from build123d import *

# Parameters (mm, degrees)
F1_DEPTH = 3.175
F3_DEPTH = 12.7
F5_R     = 1.27
F7_DEPTH = 38.1
F9_DEPTH = 57.1826710194


# Not quite as in the source:
# - a length typed as a fraction of an inch, garbled in the dataset ("3 / 203.2 mm" for 3/8 in), is restored


with BuildPart() as f1:
    # F0 (on Top) → F1 (new body)
    with BuildSketch(Plane.XY):
        Polygon((-63.5, -25.4), (63.5, -12.7), (63.5, 12.7), (-63.5, 25.4), align=None)
    extrude(amount=F1_DEPTH)

    # F2 (on Top) → F3 (join)
    with BuildSketch(Plane.XY):
        Polygon((-63.5, -25.4), (-63.5, -28.5908355097), (63.8159243079, -15.8592430789), (63.5, -12.7), align=None)
    extrude(amount=F3_DEPTH)

    # F4: F1 across plane


with BuildPart() as f1_1:
    add(f1.part)
    add(f1.part.mirror(Plane.XZ))

    # F5
    f5_edges = [f1_1.edges().sort_by_distance(p)[0] for p in [
        (0, -19.05, 3.175),
        (0, 19.05, 3.175),
    ]]
    fillet(f5_edges, radius=F5_R)

    # F6 (on face) → F7 (join)
    with BuildSketch(Plane(origin=(-63.5, 0, 0), x_dir=(0, -1, 0), z_dir=(-1, 0, 0))):
        Polygon((-25.4, 12.7), (-28.5908355097, 12.7), (-28.5908355097, 0), (-25.4, 0), (-25.4, 4.445), align=None)
        Polygon((25.4, 4.445), (25.4, 0), (28.5908355097, 0), (28.5908355097, 12.7), (25.4, 12.7), align=None)
    extrude(amount=F7_DEPTH)

    # F8 (on face) → F9 (cut, through all)
    with BuildSketch(Plane.XZ.offset(28.5908355097)):
        with BuildLine():
            Line((-92.075, 3.175), (-92.075, 9.525))
            ThreePointArc((-92.075, 9.525), (-95.25, 6.35), (-92.075, 3.175))
        make_face()
        with BuildLine():
            ThreePointArc((-88.9, 6.35), (-89.8299359697, 8.5950640303), (-92.075, 9.525))
            Line((-92.075, 9.525), (-92.075, 3.175))
            ThreePointArc((-92.075, 3.175), (-89.8299359697, 4.1049359697), (-88.9, 6.35))
        make_face()
    extrude(amount=-F9_DEPTH, mode=Mode.SUBTRACT)


solid = f1_1.part
Input: part model. Units: mm. Frame: model coordinates. A direction names the side the tool comes from. Give positions to 0.01 mm unless a question says otherwise; leave off trailing zeros. Order: outer loops, then holes, each group sorted by start corner. A loop starts at its lowest first (then second) coordinate and runs counter-clockwise, first axis right, second up. Notation, with made-up numbers: (-9.5, -5.75) - (-4.5, -5.75) arc R11 cw to (-4.5, 10.25) - close; hole circle Ø7 at (18.25, 41.25). An arc over 180 degrees is marked (long way). Answer as a JSON object with one key per item and string values. Group by question number.
Q1. Line query: probe 1 along Y at (x, z) = (12, 11.5); probe 2 along Y at (x, z) = (54.5, 6); probe 3 along Z at (x, y) = (1, 13) (3 decimals). Output: solid intervals per line, ascending.
Q2. Set-up query: faces 5 (the face through (63.66, 14.3, 6.26)), 6 (the face through (0.915, -18.575, 3.537)), 7 (the face through (-82, 25.4, 6)). Return all of +Z, -Z, +X, -X, +Y, -Y with unobstructed straight access to the full face (end or side cutting, diameter ignored); none if empty.
Q3. Cut plane A-A, the plane y = 3. Output: boundary loops of the cut face in (x, z) (3 decimals), then the cut area to 3 significant figures.
Q4. Mould query, pull axis Y, two halves, no side actions, for faces 1 (the face through (-101.6, -27, 6)), 2 (the face through (0.89, -18.96, 8.51)), 3 (the face through (-82, 28.591, 6)), 4 (the face through (-63.5, 0, 1)). Classes: pulls with the +Y half, pulls with the -Y half, needs draft (parallel to the pull), parting line crosses it, or undercut.
Q5. First-contact query: pin 1 Ø3.5 at (y, z) = (-11, 1.5) entering from -X; pin 2 Ø3.5 at (y, z) = (-1.5, 2.5) entering from +X. Flat tips, straight axial feed; report the tip coordinate or a pass-through.
Results:
{
 "1": {"probe 1": "-21.04 to -17.85, 17.85 to 21.04", "probe 2": "-16.79 to -13.6, 13.6 to 16.79", "probe 3": "0 to 3.175"},
 "2": {"face 5": "+Z, -Z, +X", "face 6": "+Z, -X", "face 7": "+Z, -Z, -X"},
 "3": {"outline": "(-63.5, 0) - (63.5, 0) - (63.5, 3.175) - (-63.5, 3.175) - close", "area": "403 mm^2"},
 "4": {"face 1": "needs draft", "face 2": "undercut", "face 3": "pulls with the +Y half", "face 4": "undercut"},
 "5": {"pin 1": "x = -63.5", "pin 2": "x = 63.5"}
}
